Here's how the part is built. I have some questions about the finished solid (model axes, mm). Round coordinates to 2 decimals unless told otherwise and drop trailing zeros. Order: outer loops, then holes, each group sorted by start corner. A loop starts at its lowest first (then second) coordinate and runs counter-clockwise, first axis right, second up. Notation, with made-up numbers: M 38.5,20.25 L 69.5,20.25 A14 ccw 69.5,45.25 Z; hole C 70.25,66 d3. An arc over 180 degrees is marked long. Write item = value, one per line. Start each with the question number.
Item 1: We'd pull the mould along X, two halves only. Please class faces 1 (the face through (5.6, 48.31, 17.79)), 2 (the face through (-10, 0, -11)), 3 (the face through (-5.611, 49.3, 13.533)): pulls with the +X half, pulls with the -X half, needs draft (parallel to the pull), parting line crosses it, or undercut.
Item 2: I want a section at A-A, the plane x = 0. List the corners of the cut face in (y, z) for me.
Item 3: I'm going to push flat-ended pins straight in: P1, Ø4, axis at x = 11, y = 49, coming from the +Z side; P2, Ø3, axis at x = -7, y = 80, coming from the -Z side; P3, Ø1.5, axis at y = 70, z = -10, coming from the +X side. Where does each tip first touch, or does it pass through?
Item 4: I want a section at B-B, the plane z = 0. List the corners of the cut face in (x, y) for me.
Item 5: I want a section at C-C, the plane y = 81.5. List the corners of the cut face in (x, z) for me, plus the area to 3 significant figures.
Item 6: Please list where these lines run through material, in increasing order: L1, parallel to X at y = 24.5, z = 0; L2, parallel to Z at x = -10.5, y = 53; L3, parallel to Z at x = 1, y = 22.
```python
from build123d import *

# Parameters (mm, degrees)
SKETCH1_R                       = 18.65
SKETCH1_R_2                     = 14.65
BOSS_EXTRUDE1_DEPTH             = 100
BOSS_EXTRUDE2_REACH             = 110.347
BOSS_EXTRUDE2_END_RADIUS        = 18.65
SKETCH3_W                       = 7.5
SKETCH3_H                       = 7.5
BOSS_EXTRUDE2_DIRECTION_2_DEPTH = 0.35
BOSS_EXTRUDE3_REACH             = 110.468
BOSS_EXTRUDE3_END_RADIUS        = 18.65
SKETCH4_W                       = 7.5
SKETCH4_H                       = 7.5
BOSS_EXTRUDE3_DIRECTION_2_DEPTH = 0.35
CHAMFER1_SIZE                   = 2


with BuildPart() as part:
    # Sketch1 → Boss-Extrude1 (new body)
    with BuildSketch(Plane(origin=(0, 0, 0), x_dir=(1, 0, 0), z_dir=(0, 1, 0))):
        with Locations(Location((0, 0, 0), (0, 0, 270))):
            Circle(SKETCH1_R)
        with Locations(Location((0, 0, 0), (0, 0, 270))):
            Circle(SKETCH1_R_2, mode=Mode.SUBTRACT)
    extrude(amount=BOSS_EXTRUDE1_DEPTH)

    # Boss-Extrude2: up to this cylinder (the profile starts outside it)
    boss_extrude2_end = Plane(origin=(0, 22.5, 0), z_dir=(0, -1, 0)) * Cylinder(BOSS_EXTRUDE2_END_RADIUS, 293.994, mode=Mode.PRIVATE)
    # Sketch3 → Boss-Extrude2 (add, up to the surface)
    with BuildSketch(Plane.XY.offset(18.65), mode=Mode.PRIVATE) as boss_extrude2_sk1:
        with Locations((0, 5)):
            Rectangle(SKETCH3_W, SKETCH3_H)
    boss_extrude2_tool1 = extrude(boss_extrude2_sk1.sketch, amount=-BOSS_EXTRUDE2_REACH, mode=Mode.PRIVATE) - boss_extrude2_end
    add(boss_extrude2_tool1.solids().sort_by_distance((0, 5, 18.65))[0])
    add(boss_extrude2_tool1.solids().sort_by_distance((0, 5, 18.65))[1])
    # Sketch3 → Boss-Extrude2 (add, up to the surface)
    with BuildSketch(Plane.XY.offset(18.65), mode=Mode.PRIVATE) as boss_extrude2_sk2:
        with Locations((0, 40)):
            Rectangle(SKETCH3_W, SKETCH3_H)
    boss_extrude2_tool2 = extrude(boss_extrude2_sk2.sketch, amount=-BOSS_EXTRUDE2_REACH, mode=Mode.PRIVATE) - boss_extrude2_end
    add(boss_extrude2_tool2.solids().sort_by_distance((0, 40, 18.65))[0])
    add(boss_extrude2_tool2.solids().sort_by_distance((0, 40, 18.65))[1])

    # Sketch3 → Boss-Extrude2 direction 2 (add)
    with BuildSketch(Plane.XY.offset(18.65)):
        with Locations((0, 5)):
            Rectangle(SKETCH3_W, SKETCH3_H)
        with Locations((0, 40)):
            Rectangle(SKETCH3_W, SKETCH3_H)
    extrude(amount=BOSS_EXTRUDE2_DIRECTION_2_DEPTH)

    # Boss-Extrude3: up to this cylinder (the profile starts outside it)
    boss_extrude3_end = Plane(origin=(0, 40, 0), z_dir=(0, -1, 0)) * Cylinder(BOSS_EXTRUDE3_END_RADIUS, 259.236, mode=Mode.PRIVATE)
    # Sketch4 → Boss-Extrude3 (add, up to the surface)
    with BuildSketch(Plane(origin=(0, 0, -18.65), x_dir=(-1, 0, 0), z_dir=(0, 0, -1)), mode=Mode.PRIVATE) as boss_extrude3_sk1:
        with Locations((0, 40)):
            Rectangle(SKETCH4_W, SKETCH4_H)
    boss_extrude3_tool1 = extrude(boss_extrude3_sk1.sketch, amount=-BOSS_EXTRUDE3_REACH, mode=Mode.PRIVATE) - boss_extrude3_end
    add(boss_extrude3_tool1.solids().sort_by_distance((0, 40, -18.65))[0])
    add(boss_extrude3_tool1.solids().sort_by_distance((0, 40, -18.65))[1])

    # Sketch4 → Boss-Extrude3 direction 2 (add)
    with BuildSketch(Plane(origin=(0, 0, -18.65), x_dir=(-1, 0, 0), z_dir=(0, 0, -1))):
        with Locations((0, 40)):
            Rectangle(SKETCH4_W, SKETCH4_H)
    extrude(amount=BOSS_EXTRUDE3_DIRECTION_2_DEPTH)

    # Chamfer1
    chamfer1_edges = [part.edges().sort_by_distance(p)[0] for p in [
        (0, 100, -18.65),
    ]]
    chamfer(chamfer1_edges, length=CHAMFER1_SIZE)


solid = part.part
```
Filled in:
q1.face_1 = parting line crosses it
q1.face_2 = needs draft
q1.face_3 = undercut
q2.outline = M 0,-18.65 L 36.25,-18.65 L 36.25,-19 L 43.75,-19 L 43.75,-18.65 L 98,-18.65 L 100,-16.65 L 100,-14.65 L 0,-14.65 Z; M 0,14.65 L 100,14.65 L 100,16.65 L 98,18.65 L 43.75,18.65 L 43.75,19 L 36.25,19 L 36.25,18.65 L 8.75,18.65 L 8.75,19 L 1.25,19 L 1.25,18.65 L 0,18.65 Z
q3.P1 = 16.33
q3.P2 = -17.82
q3.P3 = 16.19
q4.outline = M -18.65,0 L -14.65,0 L -14.65,100 L -16.65,100 L -18.65,98 Z; M 14.65,0 L 18.65,0 L 18.65,98 L 16.65,100 L 14.65,100 Z
q5.outline = C 0,0 d37.3; hole C 0,0 d29.3
q5.area = 418 mm^2
q6.L1 = -18.65 to -14.65, 14.65 to 18.65
q6.L2 = -15.41 to -10.22, 10.22 to 15.41
q6.L3 = -18.62 to -14.62, 14.62 to 18.62
